The figure shows three views and two pictorial views of one solid part (mm, origin at its lowest corner). Answer the questions. Round coordinates to 2 decimals unless told otherwise and drop trailing zeros. Write each loop counter-clockwise with the first axis right and the second up, starting at its lowest first coordinate (ties: lowest second). Pieces come first, ordered by that corner, then holes.
Item 1: Find section A-A on z = 20. Give the vertices of the cut face in (x, y), then the cut area to 4 significant figures.
Item 2: Find section C-C on y = 0.65. Give the vertices of the cut face in (x, z).
Item 3: Find the intervals of material crossed by probe 1 along X at (y, z) = (0.7, 20); probe 2 along X at (y, z) = (0.3, 14.5), in increasing order.
Item 4: Find section B-B on x = 20. Give the vertices of the cut face in (y, z).
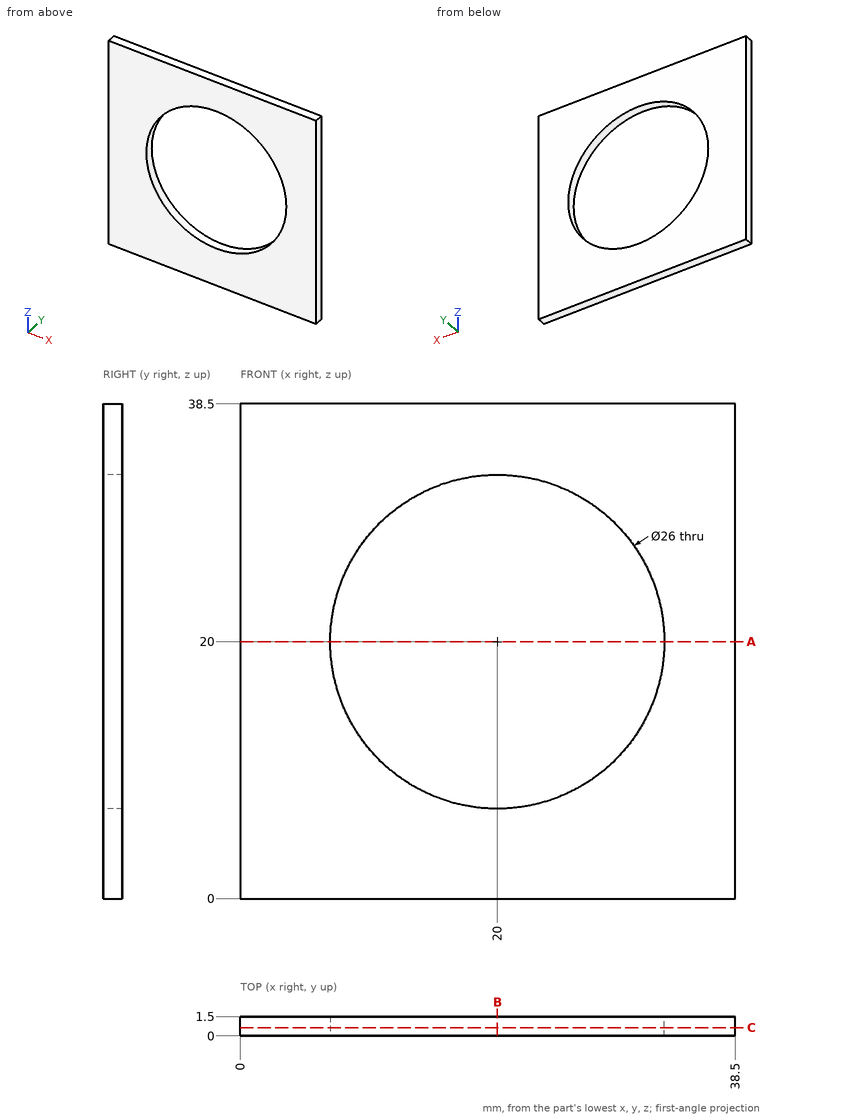
Check values:
1. outline: (0, 0) - (7, 0) - (7, 1.5) - (0, 1.5) - close; (33, 0) - (38.5, 0) - (38.5, 1.5) - (33, 1.5) - close
1. area: 18.75 mm2
2. outline: (0, 0) - (38.5, 0) - (38.5, 38.5) - (0, 38.5) - close; hole circle Ø26 at (20, 20)
3. probe 1: x = 0 to 7, 33 to 38.5
3. probe 2: x = 0 to 8.22, 31.78 to 38.5
4. outline: (0, 0) - (1.5, 0) - (1.5, 7) - (0, 7) - close; (0, 33) - (1.5, 33) - (1.5, 38.5) - (0, 38.5) - close
